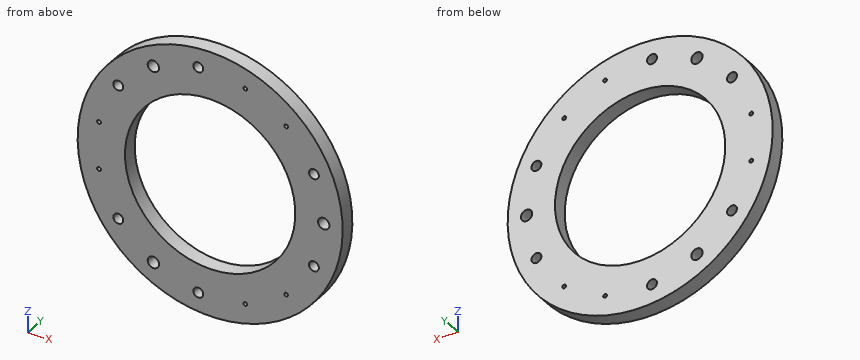
Autodesk Inventor part; units mm, degrees
ref_plane "YZ Plane" through (0, 0, 0) normal (1, 0, 0) x (0, 1, 0)
ref_plane "XZ Plane" through (0, 0, 0) normal (0, 1, 0) x (-1, 0, 0)
ref_plane "XY Plane" through (0, 0, 0) normal (0, 0, 1) x (1, 0, 0)
sketch "Sketch1" plane through (0, 0, 0) normal (1, 0, 0) x (0, 1, 0)
  line L0 (0, 22.5) -> (4, 22.5)
  line L1 (4, 22.5) -> (4, 35)
  line L2 (4, 35) -> (0, 35)
  line L3 (0, 35) -> (0, 22.5)
  line L4 (-0.8, 0) -> (4.8, 0)
  point P0 (0, 0)
  dimension "d0" = 22.5
  dimension "d1" = 35
  dimension "d2" = 4
revolve "Revolution1" add sketch "Sketch1" angle 360 about axis through (0, -10, 0) along (0, 1, 0)
sketch "Sketch2" plane through (0, 4, 0) normal (0, 1, 0) x (1, 0, 0)
  point P0 (0, 0)
  point P1 (30, 0)
  dimension "d5" = 30
hole "Hole1" at (30, 4, 0) direction (0, -1, 0) diameter 3 end through all
pattern_circular "Circular Pattern1" count 3 over 360 about axis through (0, 2, 0) along (0, 1, 0) of "Hole1"
sketch "Sketch3" plane through (0, 4, 0) normal (0, 1, 0) x (1, 0, 0)
  circle A0 centre (0, 0) radius 30 construction
  circle A1 centre (30, 0) radius 1.5
  point P0 (27.4064, 12.2021)
  point P1 (27.4064, -12.2021)
  dimension "d16" = 60
  dimension "d18" = 24
  dimension "d20" = 24
hole "Hole2" at (27.4064, 4, -12.2021) at (27.4064, 4, 12.2021) direction (0, -1, 0) diameter 2.6211 end through all
pattern_circular "Circular Pattern2" count 3 over 360 about axis through (0, 2, 0) along (0, 1, 0) of "Hole2"
sketch "Sketch4" plane through (0, 4, 0) normal (0, 1, 0) x (1, 0, 0)
  circle A0 centre (0, 0) radius 30 construction
  circle A1 centre (27.4064, -12.2021) radius 1.3106
  circle A2 centre (27.4064, 12.2021) radius 1.3106
  point P0 (20.0739, -22.2943)
  point P1 (20.0739, 22.2943)
  dimension "d31" = 60
  dimension "d34" = 24
  dimension "d35" = 24
hole "Hole3" at (20.0739, 4, -22.2943) at (20.0739, 4, 22.2943) direction (0, -1, 0) diameter 1 end through all
pattern_circular "Circular Pattern3" count 3 over 360 about axis through (0, 2, 0) along (0, 1, 0) of "Hole3"
properties part number "CentralRing-2023-1" material "Copper"
Geometry: final body of the model. Coordinates: model frame, mm. Give positions to 0.01 mm unless a question says otherwise; leave off trailing zeros. Write each loop counter-clockwise with the first axis right and the second up, starting at its lowest first coordinate (ties: lowest second). Pieces come first, ordered by that corner, then holes. Notation, with made-up numbers: (63, -0.75) -> (93, -0.75) arc R21 ccw to (93, 24.25) -> close; hole circle Ø8 at (51.25, -39.5). An arc over 180 degrees is marked (long way). Answer in a Markdown table with one row per item.
(1) Section query B-B on z = 0. Return loops of the section in (x, y), then the cut area to 3 significant figures.
Answers below:
| item | result |
|---|---|
| outline | (-35, 0) -> (-22.5, 0) -> (-22.5, 4) -> (-35, 4) -> close; (22.5, 0) -> (28.5, 0) -> (28.5, 4) -> (22.5, 4) -> close; (31.5, 0) -> (35, 0) -> (35, 4) -> (31.5, 4) -> close |
| area | 88.0 mm^2 |
(2) Section query C-C on y = 0.7. State how many separate pieces and enclosed holes the cut face has, then the cut area to 3 significant figures.
Answers below:
| item | result |
|---|---|
| separate pieces | 1 |
| enclosed holes | 16 |
| area | 2,200 mm^2 |
(3) Section query A-A on x = 0. Return loops of the section in (y, z), then the cut area to 3 significant figures.
Answers below:
| item | result |
|---|---|
| outline | (0, -35) -> (4, -35) -> (4, -22.5) -> (0, -22.5) -> close; (0, 22.5) -> (4, 22.5) -> (4, 35) -> (0, 35) -> close |
| area | 100 mm^2 |
(4) Section query D-D on z = -21. Return loops of the section in (x, y).
Answers below:
| item | result |
|---|---|
| outline | (-28, 0) -> (-8.08, 0) -> (-8.08, 4) -> (-28, 4) -> close; (8.08, 0) -> (28, 0) -> (28, 4) -> (8.08, 4) -> close |
(5) Pin query (flat end, axial travel): pin 1 (1.5 mm diameter, centred on y = 2, z = 24, fed in from +X). Return the tip coordinate at first contact, or that it passes through.
Answers below:
| item | result |
|---|---|
| pin 1 | x = 26.16 |
(6) Ray query, line 1 along X through (y, z) = (2.4, 0); line 2 along X through (y, z) = (2.4, -1); line 3 along X through (y, z) = (2.5, 19.5). Return the intervals inside material, ascending. Write a range as [from, to].
Answers below:
| item | result |
|---|---|
| line 1 | [-35, -22.5], [22.5, 28.5], [31.5, 35] |
| line 2 | [-34.99, -22.48], [22.48, 28.88], [31.12, 34.99] |
| line 3 | [-29.06, -11.22], [11.22, 29.06] |
